The model under review builds one solid part; all positions refer to its coordinate system, in mm. A direction names the side the tool comes from. Coordinates: 2 decimals unless noted, no trailing zeros. Write each loop counter-clockwise with the first axis right and the second up, starting at its lowest first coordinate (ties: lowest second). Pieces come first, ordered by that corner, then holes. Notation, with made-up numbers: (-2, 48.25) -> (9, 48.25) arc R25 ccw to (9, 83.25) -> close; hole circle Ø7 at (1, 63). An arc over 180 degrees is marked (long way). Write each question's results on one line, items separated by ' | '.
```python
from build123d import *

# Parameters (mm, degrees)
ESQUISSE1_W             = 53.3
ESQUISSE1_H             = 40
BOSS_EXTRU_1_DEPTH      = 20
ESQUISSE2_W             = 43.3
ESQUISSE2_H             = 40
ENL_V_MAT_EXTRU_1_DEPTH = 15
ESQUISSE3_R             = 1.5
ENL_V_MAT_EXTRU_2_DEPTH = 54.3


with BuildPart() as part:
    # Esquisse1 → Boss.-Extru.1 (new body)
    with BuildSketch(Plane(origin=(0, 0, 0), x_dir=(1, 0, 0), z_dir=(0, 1, 0))):
        with Locations((26.65, -20)):
            Rectangle(ESQUISSE1_W, ESQUISSE1_H)
    extrude(amount=BOSS_EXTRU_1_DEPTH)

    # Esquisse2 → Enlèv. mat.-Extru.1 (cut)
    with BuildSketch(Plane(origin=(0, 20, 0), x_dir=(1, 0, 0), z_dir=(0, 1, 0))):
        with Locations((26.65, -20)):
            Rectangle(ESQUISSE2_W, ESQUISSE2_H)
    extrude(amount=-ENL_V_MAT_EXTRU_1_DEPTH, mode=Mode.SUBTRACT)

    # Esquisse3 → Enlèv. mat.-Extru.2 (cut, through all)
    with BuildSketch(Plane(origin=(53.3, 0, 0), x_dir=(0, 0, -1), z_dir=(1, 0, 0))):
        with Locations((-30, 10)):
            Circle(ESQUISSE3_R)
        with Locations((-10, 10)):
            Circle(ESQUISSE3_R)
    extrude(amount=-ENL_V_MAT_EXTRU_2_DEPTH, mode=Mode.SUBTRACT)


solid = part.part
```
Q1. For line 1 (X direction, y = 8.5, z = 34); line 2 (Y direction, x = 3, z = 30); line 3 (Y direction, x = 23.5, z = 36), list the stretches that pass through material, from the lowest coordinate up. Write a range as from..to.
Solution:
line 1: 0..5, 48.3..53.3 | line 2: 0..8.5, 11.5..20 | line 3: 0..5
Q2. Draft analysis for pull direction Y (two halves, no side actions). For faces 1 (the flat face through (48.3, 13, 20)), 2 (the cylindrical face through (50.83, 10.07, 31.5)), 3 (the flat face through (2, 20, 20)), 4 (the cylindrical face through (2.5, 9.1, 11.2)), state which applies: pulls with the +Y half, pulls with the -Y half, needs draft (parallel to the pull), parting line crosses it, or undercut.
Solution:
face 1: needs draft | face 2: undercut | face 3: pulls with the +Y half | face 4: undercut
Q3. Add section C-C (y = 16.5). Write out the cut boundary in (x, z).
Solution:
outline: (0, 0) -> (5, 0) -> (5, 40) -> (0, 40) -> close; (48.3, 0) -> (53.3, 0) -> (53.3, 40) -> (48.3, 40) -> close
Q4. Machinability: for faces 5 (the flat face through (26, 3, 40)), 6 (the flat face through (5, 13, 20)), which of the approach directions +Z, -Z, +X, -X, +Y, -Y give a long, thin tool a straight path to every point of the face, cutting with its end or side? Answer none if there is none.
Solution:
face 5: +Z, +X, -X, +Y, -Y | face 6: +Z, -Z, +Y
Q5. Add section B-B (y = 10). Write out the cut boundary in (x, z).
Solution:
outline: (0, 0) -> (5, 0) -> (5, 8.5) -> (0, 8.5) -> close; (0, 11.5) -> (5, 11.5) -> (5, 28.5) -> (0, 28.5) -> close; (0, 31.5) -> (5, 31.5) -> (5, 40) -> (0, 40) -> close; (48.3, 0) -> (53.3, 0) -> (53.3, 8.5) -> (48.3, 8.5) -> close; (48.3, 11.5) -> (53.3, 11.5) -> (53.3, 28.5) -> (48.3, 28.5) -> close; (48.3, 31.5) -> (53.3, 31.5) -> (53.3, 40) -> (48.3, 40) -> close
Q6. Add section D-D (z = 30.5). Write out the cut boundary in (x, y).
Solution:
outline: (0, 0) -> (53.3, 0) -> (53.3, 8.59) -> (48.3, 8.59) -> (48.3, 5) -> (5, 5) -> (5, 8.59) -> (0, 8.59) -> close; (0, 11.41) -> (5, 11.41) -> (5, 20) -> (0, 20) -> close; (48.3, 11.41) -> (53.3, 11.41) -> (53.3, 20) -> (48.3, 20) -> close
Q7. Add section A-A (z = 10). Write out the cut boundary in (x, y).
Solution:
outline: (0, 0) -> (53.3, 0) -> (53.3, 8.5) -> (48.3, 8.5) -> (48.3, 5) -> (5, 5) -> (5, 8.5) -> (0, 8.5) -> close; (0, 11.5) -> (5, 11.5) -> (5, 20) -> (0, 20) -> close; (48.3, 11.5) -> (53.3, 11.5) -> (53.3, 20) -> (48.3, 20) -> close
Q8. Clearance check with flat-ended pins moving along their axes: P1, Ø2.5, axis at y = 10, z = 10, coming from the +X side; P2, Ø1, axis at x = 6.5, z = 5.5, coming from the +Y side. State where each tip first meets the part, or that it passes through.
Solution:
P1: through | P2: y = 5
